Model file for the job. Use its own axes, mm. Face numbers are marked on the shaded views. A direction names the side the tool comes from. Give positions to 0.01 mm unless a question says otherwise; leave off trailing zeros. Write each loop counter-clockwise with the first axis right and the second up, starting at its lowest first coordinate (ties: lowest second). Pieces come first, ordered by that corner, then holes. Notation, with made-up numbers: (-12, -12) - (38, -12) arc R13 ccw to (38, -4) - close; hole circle Ø5 at (-12.5, 53). An arc over 180 degrees is marked (long way). One line per item, written item: value. Start each with the question number.
(1) Probe L1, parallel to X at y = 0.5, z = 6; L2, parallel to Y at x = -34.5, z = 11; L3, parallel to Z at x = -24, y = -25. List the from-to ranges inside material, lowest first.
(2) Drop flat-ended pins along their axis: P1, Ø6.5, axis at x = 36.5, z = 30, coming from the -Y side; P2, Ø1, axis at y = -35, z = 34.5, coming from the -X side; P3, Ø4, axis at x = -10, z = 36.5, coming from the -Y side. Give the stop position or say it passes through.
(3) Cut at D-D, the plane z = 7.5. List the corners of the cut face in (x, y).
(4) 3-axis set-ups, long thin cutter, end or side, ignore diameter. For the marked faces 1, 2, 3 and 4: which of +Z, -Z, +X, -X, +Y, -Y reach the whole face in a straight line?
(5) Cut at B-B, the plane x = 0. List the corners of the cut face in (y, z).
(6) Cut at A-A, the plane y = -50. List the corners of the cut face in (x, z), and give its area (3 significant figures).
(7) Mould opens along X. For the marked faces 5, 6 and 7 say: pulls with the +X half, pulls with the -X half, needs draft (parallel to the pull), parting line crosses it, or undercut.
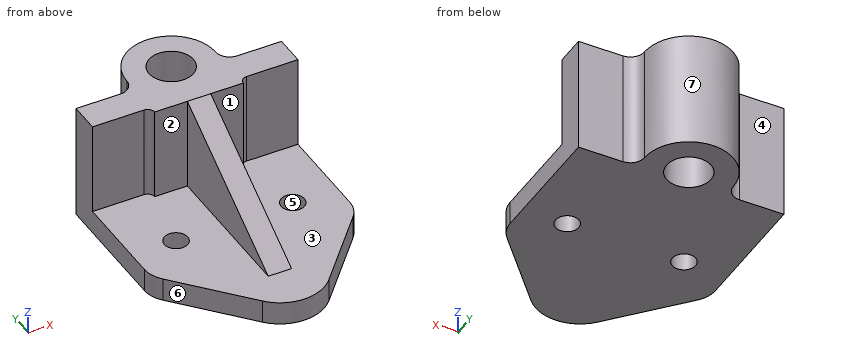
from build123d import *

# Parameters (mm, degrees)
SKETCH1_R           = 5
BOSS_EXTRUDE1_DEPTH = 10
SKETCH1_3_R         = 9.5
BOSS_EXTRUDE2_DEPTH = 50
RIB1_REACH          = 126.342
SKETCH2_WALL_W      = 326.156388182
SKETCH2_WALL_H      = 10
FILLET1_R           = 3


with BuildPart() as part:
    # Sketch1 → Boss-Extrude1 (new body)
    with BuildSketch(Plane.XY):
        with BuildLine():
            Line((-19, -19), (-44, -19))
            Line((-44, -19), (-44, -60))
            ThreePointArc((-44, -60), (-43.157361579, -64.604189335), (-40.738683164, -68.61150685))
            Line((-40.738683164, -68.61150685), (-14.233460009, -98.586048473))
            ThreePointArc((-14.233460009, -98.586048473), (0, -105), (14.233460009, -98.586048473))
            Line((14.233460009, -98.586048473), (40.738683164, -68.61150685))
            ThreePointArc((40.738683164, -68.61150685), (43.157361579, -64.604189335), (44, -60))
            Line((44, -60), (44, -19))
            Line((44, -19), (19, -19))
            Line((19, -19), (19, -22))
            Line((19, -22), (-19, -22))
            Line((-19, -22), (-19, -19))
        make_face()
        with Locations((-25, -50)):
            Circle(SKETCH1_R, mode=Mode.SUBTRACT)
        with Locations((25, -50)):
            Circle(SKETCH1_R, mode=Mode.SUBTRACT)
    extrude(amount=BOSS_EXTRUDE1_DEPTH)

    # Sketch1<3> → Boss-Extrude2 (add)
    with BuildSketch(Plane.XY):
        with BuildLine():
            Line((-25, -6), (-44, -6))
            Line((-44, -6), (-44, -19))
            Line((-44, -19), (-19, -19))
            Line((-19, -19), (-19, -22))
            Line((-19, -22), (19, -22))
            Line((19, -22), (19, -19))
            Line((19, -19), (44, -19))
            Line((44, -19), (44, -6))
            Line((44, -6), (25, -6))
            ThreePointArc((25, -6), (20.757359313, -4.242640687), (19, 0))
            ThreePointArc((19, 0), (0, 19), (-19, 0))
            ThreePointArc((-19, 0), (-20.757359313, -4.242640687), (-25, -6))
        make_face()
        Circle(SKETCH1_3_R, mode=Mode.SUBTRACT)
    extrude(amount=BOSS_EXTRUDE2_DEPTH)

    # Sketch2 wall → Rib1 (add, up to next)
    with BuildSketch(Plane(origin=(0, -54, 30), x_dir=(0, -0.847998304005, -0.529998940003), z_dir=(0, 0.529998940003, -0.847998304005)), mode=Mode.PRIVATE) as rib1_sk1:
        Rectangle(SKETCH2_WALL_W, SKETCH2_WALL_H)
    rib1_tool1 = extrude(rib1_sk1.sketch, amount=RIB1_REACH, mode=Mode.PRIVATE) - part.part
    add(rib1_tool1.solids().sort_by_distance((0, -54, 30))[0])

    # Fillet1
    fillet1_edges = [part.edges().sort_by_distance(p)[0] for p in [
        (-19, -19, 30),
        (19, -19, 30),
    ]]
    fillet(fillet1_edges, radius=FILLET1_R - 0.0001)  # a hair under: the kernel refuses the full size


solid = part.part
Answers follow:
1. L1: x = -18.99 to -9.49, 9.49 to 18.99
1. L2: y = -19 to -6
1. L3: z = 0 to 10
2. P1: stops at y = -19
2. P2: stops at x = -5
2. P3: stops at y = -22
3. outline: (-44, -60) arc R13 ccw to (-40.74, -68.61) - (-14.23, -98.59) arc R19 ccw to (14.23, -98.59) - (40.74, -68.61) arc R13 ccw to (44, -60) - (44, -6) - (25, -6) arc R6 cw to (19, 0) arc R19 ccw to (-19, 0) arc R6 cw to (-25, -6) - (-44, -6) - close; hole circle Ø10 at (-25, -50); hole circle Ø19 at (0, 0); hole circle Ø10 at (25, -50)
4. face 1: +Z, +X, -Y
4. face 2: +Z, -X, -Y
4. face 3: +Z, -Y
4. face 4: +Z, -Z, -X, +Y
5. outline: (-105, 0) - (-9.5, 0) - (-9.5, 50) - (-22, 50) - (-86, 10) - (-105, 10) - close; (9.5, 0) - (19, 0) - (19, 50) - (9.5, 50) - close
6. outline: (-44, 0) - (-30, 0) - (-30, 10) - (-44, 10) - close; (-20, 0) - (20, 0) - (20, 10) - (5, 10) - (5, 32.5) - (-5, 32.5) - (-5, 10) - (-20, 10) - close; (30, 0) - (44, 0) - (44, 10) - (30, 10) - close
6. area: 905 mm²
7. face 5: undercut
7. face 6: pulls with the -X half
7. face 7: parting line crosses it
